Part model, mm, in its own coordinate system. A direction names the side the tool comes from. Round coordinates to 2 decimals unless told otherwise and drop trailing zeros. Loops run counter-clockwise (first coordinate to the right, second up) from the corner with the lowest first, then second, coordinate; pieces in that order, holes last. Notation, with made-up numbers: (38, 85.25) -> (90, 85.25) arc R29 cw to (90, 107.25) -> close; hole circle Ø11 at (3.25, -13.75). An arc over 180 degrees is marked (long way). Use a Markdown table: item, result. Add a question column.
Item 1: Two-plate mould, pull along Z, no slides. Class faces 3 (the face through (4, 0, 3)), 4 (the face through (-2.064, 2.348, 4.393)), 5 (the face through (-9.89, 2.35, 71.86)): pulls with the +Z half, pulls with the -Z half, needs draft (parallel to the pull), parting line crosses it, or undercut.
Item 2: Flat gauge pins, fed straight in: pin 1 (1.5 mm diameter, centred on x = 41.5, z = 43.5, fed in from +Y); pin 2 (1.4 mm diameter, centred on x = 37.5, y = 2, fed in from -Z); pin 3 (1.4 mm diameter, centred on x = 31.5, y = 2.5, fed in from +Z); pin 4 (1.5 mm diameter, centred on y = 2, z = 3.5, fed in from +X). Where does each tip first touch, or does it go through?
Item 3: Cut at C-C, the plane x = -24. List the corners of the cut face in (y, z).
Item 4: Cut at D-D, the plane y = 1.9. State how many separate pieces and enclosed holes the cut face has, plus the area to 3 significant figures.
Item 5: Which spindle directions (+Z, -Z, +X, -X, +Y, -Y) get a long thin tool onto all of the face, cutting with end or side? Do faces 1 (the face through (4, 4.762, 3)), 2 (the face through (-57.626, 2.348, 4.497)). Say none if no direction does.
Item 6: Cut at A-A, the plane z = -27.5. List the corners of the cut face in (x, y), plus the area to 3 significant figures.
Item 7: Probe line 1 (X direction, y = 1.75, z = 29); line 2 (Z direction, x = 36.5, y = 4.4); line 3 (Z direction, x = -24.5, y = 1.45). List the from-to ranges inside material, lowest first. Write a range as [from, to].
Item 8: Cut at B-B, the plane x = 5.08. List the corners of the cut face in (y, z).
```python
from build123d import *

# Parameters (mm, degrees)
SKETCH1_R           = 69.05625
BOSS_EXTRUDE1_DEPTH = 4.7625


with BuildPart() as part:
    # Sketch1 → Boss-Extrude1 (new body)
    with BuildSketch(Plane(origin=(0, 0, 0), x_dir=(1, 0, 0), z_dir=(0, 1, 0))):
        with Locations((5.08, -4.445)):
            Circle(SKETCH1_R)
        with BuildLine():
            Line((2.69875, 5.08), (2.69875, 55.88))
            ThreePointArc((2.69875, 55.88), (5.08, 58.26125), (7.46125, 55.88))
            Line((7.46125, 55.88), (7.46125, 5.08))
            ThreePointArc((7.46125, 5.08), (5.08, 2.69875), (2.69875, 5.08))
        make_face(mode=Mode.SUBTRACT)
        with BuildLine():
            Line((10.131394068, 3.973990114), (46.052418552, 39.895014598))
            ThreePointArc((46.052418552, 39.895014598), (49.420014598, 39.895014598), (49.420014598, 36.527418552))
            Line((49.420014598, 36.527418552), (13.498990114, 0.606394068))
            ThreePointArc((13.498990114, 0.606394068), (10.131394068, 0.606394068), (10.131394068, 3.973990114))
        make_face(mode=Mode.SUBTRACT)
        with BuildLine():
            Line((14.605, -2.06375), (65.405, -2.06375))
            ThreePointArc((65.405, -2.06375), (67.78625, -4.445), (65.405, -6.82625))
            Line((65.405, -6.82625), (14.605, -6.82625))
            ThreePointArc((14.605, -6.82625), (12.22375, -4.445), (14.605, -2.06375))
        make_face(mode=Mode.SUBTRACT)
        with BuildLine():
            Line((13.498990114, -9.496394068), (49.420014598, -45.417418552))
            ThreePointArc((49.420014598, -45.417418552), (49.420014598, -48.785014598), (46.052418552, -48.785014598))
            Line((46.052418552, -48.785014598), (10.131394068, -12.863990114))
            ThreePointArc((10.131394068, -12.863990114), (10.131394068, -9.496394068), (13.498990114, -9.496394068))
        make_face(mode=Mode.SUBTRACT)
        with BuildLine():
            Line((7.46125, -13.97), (7.46125, -64.77))
            ThreePointArc((7.46125, -64.77), (5.08, -67.15125), (2.69875, -64.77))
            Line((2.69875, -64.77), (2.69875, -13.97))
            ThreePointArc((2.69875, -13.97), (5.08, -11.58875), (7.46125, -13.97))
        make_face(mode=Mode.SUBTRACT)
        with BuildLine():
            Line((0.028605932, -12.863990114), (-35.892418552, -48.785014598))
            ThreePointArc((-35.892418552, -48.785014598), (-39.260014598, -48.785014598), (-39.260014598, -45.417418552))
            Line((-39.260014598, -45.417418552), (-3.338990114, -9.496394068))
            ThreePointArc((-3.338990114, -9.496394068), (0.028605932, -9.496394068), (0.028605932, -12.863990114))
        make_face(mode=Mode.SUBTRACT)
        with BuildLine():
            Line((-4.445, -6.82625), (-55.245, -6.82625))
            ThreePointArc((-55.245, -6.82625), (-57.62625, -4.445), (-55.245, -2.06375))
            Line((-55.245, -2.06375), (-4.445, -2.06375))
            ThreePointArc((-4.445, -2.06375), (-2.06375, -4.445), (-4.445, -6.82625))
        make_face(mode=Mode.SUBTRACT)
        with BuildLine():
            Line((-3.338990114, 0.606394068), (-39.260014598, 36.527418552))
            ThreePointArc((-39.260014598, 36.527418552), (-39.260014598, 39.895014598), (-35.892418552, 39.895014598))
            Line((-35.892418552, 39.895014598), (0.028605932, 3.973990114))
            ThreePointArc((0.028605932, 3.973990114), (0.028605932, 0.606394068), (-3.338990114, 0.606394068))
        make_face(mode=Mode.SUBTRACT)
    extrude(amount=BOSS_EXTRUDE1_DEPTH)


solid = part.part
```
A:
| question | item | result |
|---|---|---|
| 1 | face 3 | needs draft |
| 1 | face 4 | undercut |
| 1 | face 5 | parting line crosses it |
| 2 | pin 1 | stops at y = 4.76 |
| 2 | pin 2 | stops at z = -56.9 |
| 2 | pin 3 | stops at z = 68.53 |
| 2 | pin 4 | stops at x = 74.14 |
| 3 | outline | (0, -58.19) -> (4.76, -58.19) -> (4.76, -28) -> (0, -28) -> close; (0, -21.27) -> (4.76, -21.27) -> (4.76, 2.06) -> (0, 2.06) -> close; (0, 6.83) -> (4.76, 6.83) -> (4.76, 30.16) -> (0, 30.16) -> close; (0, 36.89) -> (4.76, 36.89) -> (4.76, 67.08) -> (0, 67.08) -> close |
| 4 | separate pieces | 1 |
| 4 | enclosed holes | 8 |
| 4 | area | 12,900 mm^2 |
| 5 | face 1 | +Z, -Z, +X, -X, +Y |
| 5 | face 2 | +Y, -Y |
| 6 | outline | (-56.14, 0) -> (-30.23, 0) -> (-30.23, 4.76) -> (-56.14, 4.76) -> close; (-23.5, 0) -> (2.7, 0) -> (2.7, 4.76) -> (-23.5, 4.76) -> close; (7.46, 0) -> (33.66, 0) -> (33.66, 4.76) -> (7.46, 4.76) -> close; (40.39, 0) -> (66.3, 0) -> (66.3, 4.76) -> (40.39, 4.76) -> close |
| 6 | area | 496 mm^2 |
| 7 | line 1 | x = [-59.46, -22.84], [-16.11, 2.7], [7.46, 26.27], [33, 69.62] |
| 7 | line 2 | z = [-57.05, -30.34], [-23.61, 2.06], [6.83, 32.5], [39.23, 65.94] |
| 7 | line 3 | z = [-57.96, -28.5], [-21.77, 2.06], [6.83, 30.66], [37.39, 66.85] |
| 8 | outline | (0, -64.61) -> (4.76, -64.61) -> (4.76, -58.26) -> (0, -58.26) -> close; (0, -2.7) -> (4.76, -2.7) -> (4.76, 11.59) -> (0, 11.59) -> close; (0, 67.15) -> (4.76, 67.15) -> (4.76, 73.5) -> (0, 73.5) -> close |
